Geometry check sheet. Reference: the model listing, model coordinates, mm. Coordinates: 2 decimals unless noted, no trailing zeros. Order: outer loops, then holes, each group sorted by start corner. A loop starts at its lowest first (then second) coordinate and runs counter-clockwise, first axis right, second up. Notation, with made-up numbers: M 42.25,36 L 68.25,36 A27 ccw 68.25,67 Z; hole C 55.5,27.25 d5. An arc over 180 degrees is marked long. Use CSV: the item, a comma, the result in double quotes. Start each with the question number.
```python
from build123d import *

# Parameters (mm, degrees)
SKETCH1_R             = 6.35
BOSS_EXTRUDE1_DEPTH   = 3.175
F_4_40_TAPPED_HOLE1_D = 2.2606
CHAMFER1_SIZE         = 0.508


with BuildPart() as part:
    # Sketch1 → Boss-Extrude1 (new body)
    with BuildSketch(Plane(origin=(0, 0, 0), x_dir=(1, 0, 0), z_dir=(0, 1, 0))):
        with Locations(Location((0, 0, 0), (0, 0, 270))):
            Circle(SKETCH1_R)
    extrude(amount=BOSS_EXTRUDE1_DEPTH)

    # #4-40 Tapped Hole1 (through all)
    with Locations(Plane(origin=(0, 3.175, 0), x_dir=(1, 0, 0), z_dir=(0, 1, 0))):
        with Locations((0, 0)):
            Hole(F_4_40_TAPPED_HOLE1_D / 2)

    # Chamfer1
    chamfer1_edges = [part.edges().sort_by_distance(p)[0] for p in [
        (0, 0, -6.35),
        (0, 3.175, -6.35),
    ]]
    chamfer(chamfer1_edges, length=CHAMFER1_SIZE)


solid = part.part
```
1) Section check A-A on z = 0. Record the boundary of the cut face in (x, y) (3 decimals).
2) Gauge pin test, flat end, axial feed: P1, Ø5, axis at x = -0.5, z = 3.5, coming from the -Y side. Record the tip position at first contact, or that the pin passes through.
3) Section check B-B on x = 0. Record the boundary of the cut face in (y, z) (3 decimals).
4) Draft check along X on faces 1 (the face through (0.245, 1.565, 1.103)), 2 (the face through (0.1, 3.175, -1.4)), 3 (the face through (-3.86, 1.57, -5.04)). Enter one of: +X half, -X half, draft (parallel to the pull), parting line (faces both ways), or undercut.
5) Material ranges on line 1 along Z through (x, y) = (5.5, 2.1); line 2 along Z through (x, y) = (4, 2.95); line 3 along X through (y, z) = (0.25, 1.5), recorded low to high.
6) Section check C-C on y = 1.9. Record the boundary of the cut face in (x, z), then the cut area to 3 significant figures.
Results are:
1,outline,"M -6.35,0.508 L -5.842,0 L -1.13,0 L -1.13,3.175 L -5.842,3.175 L -6.35,2.667 Z; M 1.13,0 L 5.842,0 L 6.35,0.508 L 6.35,2.667 L 5.842,3.175 L 1.13,3.175 Z"
2,P1,"stops at y = 0"
3,outline,"M 0,-5.842 L 0.508,-6.35 L 2.667,-6.35 L 3.175,-5.842 L 3.175,-1.13 L 0,-1.13 Z; M 0,1.13 L 3.175,1.13 L 3.175,5.842 L 2.667,6.35 L 0.508,6.35 L 0,5.842 Z"
4,face 1,"undercut"
4,face 2,"draft"
4,face 3,"parting line"
5,line 1,"z = -3.17 to 3.17"
5,line 2,"z = -4.56 to 4.56"
5,line 3,"x = -5.9 to 5.9"
6,outline,"C 0,0 d12.7; hole C 0,0 d2.26"
6,area,"123 mm²"
